```python
from build123d import *

# Parameters (mm, degrees)
SKETCH1_R           = 5
BOSS_EXTRUDE2_DEPTH = 11.9
SKETCH3_R           = 10
BOSS_EXTRUDE3_DEPTH = 15.9
BOSS_EXTRUDE4_START = 10.4
SKETCH5_R           = 10
BOSS_EXTRUDE4_DEPTH = 10.4
BOSS_EXTRUDE5_START = 23
SKETCH6_R           = 5
BOSS_EXTRUDE5_DEPTH = 23
SKETCH7_R           = 10
SKETCH7_R_2         = 5
BOSS_EXTRUDE6_DEPTH = 2
BOSS_EXTRUDE7_START = 1
SKETCH8_R           = 5
BOSS_EXTRUDE7_DEPTH = 1
BOSS_EXTRUDE8_START = 5
SKETCH9_R           = 10
BOSS_EXTRUDE8_DEPTH = 5


with BuildPart() as part:
    # Sketch1 → Boss-Extrude2 (new body)
    with BuildSketch(Plane(origin=(0, 0, 0), x_dir=(1, 0, 0), z_dir=(0, 1, 0))):
        Circle(SKETCH1_R)
        with BuildLine():
            Line((-2, 6.782575695), (-2, 4.582575695))
            ThreePointArc((-2, 4.582575695), (0, 5), (2, 4.582575695))
            Line((2, 4.582575695), (2, 6.782575695))
            Line((2, 6.782575695), (-2, 6.782575695))
        make_face()
    extrude(amount=BOSS_EXTRUDE2_DEPTH)

    # Sketch3 → Boss-Extrude3 (add)
    with BuildSketch(Plane(origin=(0, 11.9, 0), x_dir=(1, 0, 0), z_dir=(0, 1, 0))):
        with Locations(Location((0, 0, 0), (0, 0, 270))):
            Circle(SKETCH3_R)
    extrude(amount=BOSS_EXTRUDE3_DEPTH)

    # Sketch5 → Boss-Extrude4 (add)
    with BuildSketch(Plane.XZ.offset(BOSS_EXTRUDE4_START)):
        with Locations(Location((0, 0, 0), (0, 0, 90))):
            Circle(SKETCH5_R)
    extrude(amount=-BOSS_EXTRUDE4_DEPTH)

    # Sketch6 → Boss-Extrude5 (add)
    with BuildSketch(Plane.XZ.offset(10.4).offset(BOSS_EXTRUDE5_START)):
        with Locations(Location((0, 0, 0), (0, 0, 270))):
            Circle(SKETCH6_R)
    extrude(amount=-BOSS_EXTRUDE5_DEPTH)

    # Sketch7 → Boss-Extrude6 (add)
    with BuildSketch(Plane.XZ.offset(33.4)):
        with Locations(Location((0, 0, 0), (0, 0, 90))):
            Circle(SKETCH7_R)
        with Locations(Location((0, 0, 0), (0, 0, 270))):
            Circle(SKETCH7_R_2, mode=Mode.SUBTRACT)
    extrude(amount=-BOSS_EXTRUDE6_DEPTH)

    # Sketch8 → Boss-Extrude7 (add)
    with BuildSketch(Plane.XZ.offset(33.4).offset(BOSS_EXTRUDE7_START)):
        with Locations(Location((0, 0, 0), (0, 0, 270))):
            Circle(SKETCH8_R)
        with BuildLine():
            Line((-3, 8.6), (-3, 4))
            ThreePointArc((-3, 4), (0, 5), (3, 4))
            Line((3, 4), (3, 8.6))
            Line((3, 8.6), (-3, 8.6))
        make_face()
        with BuildLine():
            ThreePointArc((3, -4), (0, -5), (-3, -4))
            Line((-3, -4), (-3, -8.6))
            Line((-3, -8.6), (3, -8.6))
            Line((3, -8.6), (3, -4))
        make_face()
    extrude(amount=-BOSS_EXTRUDE7_DEPTH)

    # Sketch9 → Boss-Extrude8 (add)
    with BuildSketch(Plane(origin=(0, -34.4, 0), x_dir=(-1, 0, 0), z_dir=(0, -1, 0)).offset(BOSS_EXTRUDE8_START)):
        with Locations(Location((0, 0, 0), (0, 0, 270))):
            Circle(SKETCH9_R)
    extrude(amount=-BOSS_EXTRUDE8_DEPTH)


solid = part.part
```
Could you check a few things on this model? Use its own coordinates, in mm. A direction names the side the tool comes from. Give positions to 0.01 mm unless a question says otherwise; leave off trailing zeros. Loops run counter-clockwise (first coordinate to the right, second up) from the corner with the lowest first, then second, coordinate; pieces in that order, holes last. Notation, with made-up numbers: (60, -26.75) - (110, -26.75) arc R30 cw to (110, 2.25) - close; hole circle Ø1 at (70, 36). An arc over 180 degrees is marked (long way). Answer in a Markdown table with one row per item. Add a question column.
Q1. Which directions (+Z, -Z, +X, -X, +Y, -Y) give clear straight access to the entire face, cutting with the end or side of a thin tool? Please do faces 4 (the face through (0, 6, -6.783)), 5 (the face through (2, 6, -6)), 6 (the face through (-5, -34, 0)), 7 (the face through (5, -34, 0)), 8 (the face through (-5, -31.4, 2)).
Q2. Please list where these lines run through material, in increasing order: L1, parallel to Y at x = 8.5, z = -4; L2, parallel to Y at x = 1.5, z = 6; L3, parallel to Y at x = -1.5, z = -6.25. Write a range as from..to.
Q3. If we section it at D-D (y = 13): List the corners of the cut face in (x, z) for me.
Q4. If we section it at C-C (z = 0): List the corners of the cut face in (x, y) for me.
Q5. For pin 1 (1 mm diameter, centred on y = -8, z = -1.5, fed in from +X); pin 2 (4 mm diameter, centred on x = 4, y = -0.5, fed in from -Z); pin 3 (1.1 mm diameter, centred on x = -1, y = -34, fed in from -Z), each with a flat end and sliding along its axis, tell me the tip position at first contact or that it passes through.
Q6. We'd pull the mould along Y, two halves only. Please class faces 1 (the face through (-9.76, 19.74, -2.17)), 2 (the face through (0, 27.8, 0)), 3 (the face through (-2, 6, -6)): +Y half, -Y half, draft (parallel to the pull), parting line (faces both ways), or undercut.
Q7. If we section it at B-B (x = 8.5): List the corners of the cut face in (y, z) for me.
Q8. If we section it at A-A (z = -8): List the corners of the cut face in (x, y) for me, plus the area to 3 significant figures.
The answers:
| question | item | result |
|---|---|---|
| 1 | face 4 | -Z, +X, -X |
| 1 | face 5 | -Z, +X |
| 1 | face 6 | -X |
| 1 | face 7 | +X |
| 1 | face 8 | none |
| 2 | L1 | y = -39.4..-34.4, -33.4..-31.4, -10.4..0, 11.9..27.8 |
| 2 | L2 | y = -39.4..-31.4, -10.4..0, 11.9..27.8 |
| 2 | L3 | y = -39.4..-31.4, -10.4..27.8 |
| 3 | outline | circle Ø20 at (0, 0) |
| 4 | outline | (-10, -39.4) - (10, -39.4) - (10, -34.4) - (5, -34.4) - (5, -33.4) - (10, -33.4) - (10, -31.4) - (5, -31.4) - (5, -10.4) - (10, -10.4) - (10, 0) - (5, 0) - (5, 11.9) - (10, 11.9) - (10, 27.8) - (-10, 27.8) - (-10, 11.9) - (-5, 11.9) - (-5, 0) - (-10, 0) - (-10, -10.4) - (-5, -10.4) - (-5, -31.4) - (-10, -31.4) - (-10, -33.4) - (-5, -33.4) - (-5, -34.4) - (-10, -34.4) - close |
| 5 | pin 1 | stops at x = 9.95 |
| 5 | pin 2 | stops at z = -9.8 |
| 5 | pin 3 | stops at z = -9.98 |
| 6 | face 1 | draft |
| 6 | face 2 | +Y half |
| 6 | face 3 | undercut |
| 7 | outline | (-39.4, -5.27) - (-34.4, -5.27) - (-34.4, 5.27) - (-39.4, 5.27) - close; (-33.4, -5.27) - (-31.4, -5.27) - (-31.4, 5.27) - (-33.4, 5.27) - close; (-10.4, -5.27) - (0, -5.27) - (0, 5.27) - (-10.4, 5.27) - close; (11.9, -5.27) - (27.8, -5.27) - (27.8, 5.27) - (11.9, 5.27) - close |
| 8 | outline | (-6, -39.4) - (6, -39.4) - (6, -34.4) - (3, -34.4) - (3, -33.4) - (6, -33.4) - (6, -31.4) - (-6, -31.4) - (-6, -33.4) - (-3, -33.4) - (-3, -34.4) - (-6, -34.4) - close; (-6, -10.4) - (6, -10.4) - (6, 0) - (-6, 0) - close; (-6, 11.9) - (6, 11.9) - (6, 27.8) - (-6, 27.8) - close |
| 8 | area | 406 mm^2 |
